Autodesk Fusion 360 part; units mm, degrees
sketch "Sketch1" plane through (0, 0, 0) normal (0, 1, 0) x (1, 0, 0)
  line L0 (0, 0) -> (52.0778, 0)
  line L1 (52.0778, 0) -> (59.2706, -16)
  line L2 (59.2706, -16) -> (71.3705, -16)
  line L3 (0, 3) -> (54.0184, 3)
  line L4 (54.0184, 3) -> (61.2112, -13)
  line L5 (61.2112, -13) -> (71.3705, -13)
  line L6 (71.3705, -16) -> (71.3705, -13)
  line L7 (52.0778, 0) -> (54.0184, 3)
  dimension "d1" = -3
revolve "Revolve1" add sketch "Sketch1" angle 360 about axis through (0, 0, 1.75) along (0, 0, 1)
chamfer "Chamfer1" distance 2 distance2 7 1 edges at (-48.5536, -18.8321, 0) measured on face at (53.1063, -5.3141, -2)
chamfer "Chamfer2" distance 2 distance2 2 1 edges at (-66.5407, -25.8087, 16) measured on face at (67.0715, -3.5457, 16)
chamfer "Chamfer3" distance 8 distance2 8 1 edges at (-57.0689, -22.1349, 13) measured on face at (67.7183, -3.5457, 13)
Source: CAD feature listing. Evaluate the final solid. Frame: model axes, mm. Round coordinates to 2 decimals unless told otherwise and drop trailing zeros. Use a Markdown table: item, result. Add a question column.
1. Contact query for flat-ended pins moving along their axis: pin 1 (10 mm diameter, centred on x = -36.5, z = 9, fed in from +Y); pin 2 (10 mm diameter, centred on x = -54.5, z = 8.5, fed in from -Y); pin 3 (1.5 mm diameter, centred on x = -19, z = 7, fed in from -Y). Output: stop coordinate, or through.
2. Ray query, line 1 along Y through (x, z) = (15, 6); line 2 along X through (y, z) = (-14, 4); line 3 along Y through (x, z) = (-46, 4). Return the intervals inside material, ascending. Write a range as [from, to].
3. Pull-direction query (Y, two-part tool) for faces 1 (the cylindrical face through (68.075, -21.438, 13.493)), 2 (the conical face through (-11.97, -53.905, 6.986)), 3 (the flat face through (-58.5, 37.3, 13)); classes: +Y half, -Y half, draft (parallel to the pull), parting line (faces both ways), or undercut.
Solution:
| question | item | result |
|---|---|---|
| 1 | pin 1 | stops at y = 63.02 |
| 1 | pin 2 | stops at y = -48.54 |
| 1 | pin 3 | stops at y = -58.09 |
| 2 | line 1 | y = [-56.43, -52.77], [52.77, 56.43] |
| 2 | line 2 | x = [-55.42, -52.59], [52.59, 55.42] |
| 2 | line 3 | y = [-33.94, -29.08], [29.08, 33.94] |
| 3 | face 1 | parting line |
| 3 | face 2 | undercut |
| 3 | face 3 | draft |
